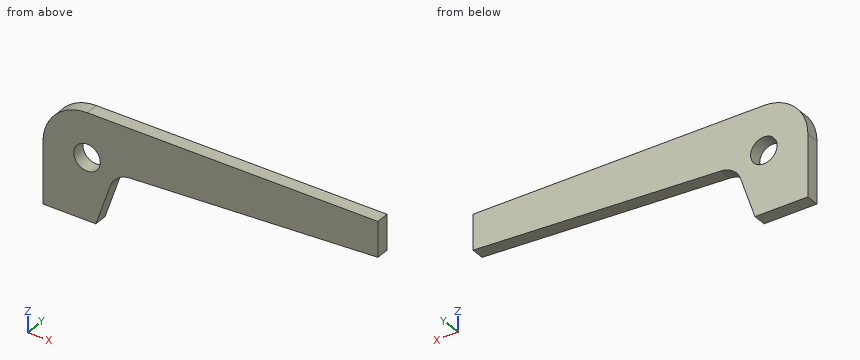
```python
from build123d import *

# Parameters (mm, degrees)
F1_DEPTH = 2.38125
F2_R     = 2.38125
F3_DEPTH = 2.38225


with BuildPart() as f1:
    # F0 (on Front) → F1 (new body)
    with BuildSketch(Plane.XZ):
        with BuildLine():
            Line((66.909325, 27.498861), (14.534525, 27.498861))
            ThreePointArc((14.534525, 27.498861), (8.912885, 25.170302), (6.584325, 19.548661))
            Line((6.584325, 19.548661), (6.584325, 8.448861))
            Line((6.584325, 8.448861), (16.109325, 8.448861))
            Line((16.109325, 8.448861), (18.69467, 16.075104))
            ThreePointArc((18.69467, 16.075104), (20.058081, 17.966739), (22.247746, 18.768327))
            Line((22.247746, 18.768327), (66.909325, 21.148861))
            Line((66.909325, 21.148861), (66.909325, 27.498861))
        make_face()
    extrude(amount=F1_DEPTH)

    # F2 (on face) → F3 (cut, through all)
    with BuildSketch(Plane.XZ.offset(2.38125)):
        with Locations((14.521825, 19.561361)):
            Circle(F2_R)
    extrude(amount=-F3_DEPTH, mode=Mode.SUBTRACT)


solid = f1.part
```
Geometry check sheet. Reference: the model listing, model coordinates, mm. Round coordinates to 2 decimals unless told otherwise and drop trailing zeros. Loops run counter-clockwise (first coordinate to the right, second up) from the corner with the lowest first, then second, coordinate; pieces in that order, holes last. Notation, with made-up numbers: (65, 57) -> (107, 57) arc R11 ccw to (107, 77) -> close; hole circle Ø1 at (87.25, 1). An arc over 180 degrees is marked (long way). Use a Markdown table: item, result.
(1) Sectioned sample at B-B (x = 38.5). Enter the section's corners in (y, z).
Calculated:
| item | result |
|---|---|
| outline | (-2.38, 19.63) -> (0, 19.63) -> (0, 27.5) -> (-2.38, 27.5) -> close |
(2) Sectioned sample at C-C (z = 23.5). Enter the section's corners in (x, y).
Calculated:
| item | result |
|---|---|
| outline | (7.64, -2.38) -> (66.91, -2.38) -> (66.91, 0) -> (7.64, 0) -> close |
(3) Go/stop test with a flat-tipped pin: P1, Ø5.5, axis at x = 14.52, z = 19.56, coming from the +Y side. Record where the tip stops, or that it passes through.
Calculated:
| item | result |
|---|---|
| P1 | y = 0 |
(4) Sectioned sample at A-A (y = -0.8). Enter the section's corners in (x, z).
Calculated:
| item | result |
|---|---|
| outline | (6.58, 8.45) -> (16.11, 8.45) -> (18.69, 16.08) arc R3.98 cw to (22.25, 18.77) -> (66.91, 21.15) -> (66.91, 27.5) -> (14.53, 27.5) arc R7.95 ccw to (6.58, 19.55) -> close; hole circle Ø4.76 at (14.52, 19.56) |
(5) Scan lines: probe 1 along Z at (x, y) = (15.5, -1.7); probe 2 along Z at (x, y) = (62.5, -1.1); probe 3 along Z at (x, y) = (37, -0.75). Record each from-to range of solid material in increasing order.
Calculated:
| item | result |
|---|---|
| probe 1 | 8.45 to 17.39, 21.73 to 27.5 |
| probe 2 | 20.91 to 27.5 |
| probe 3 | 19.55 to 27.5 |
